Check sheet for the modelled part. Datum: model origin and axes. Units: mm. Give positions to 0.01 mm unless a question says otherwise; leave off trailing zeros. Order: outer loops, then holes, each group sorted by start corner. A loop starts at its lowest first (then second) coordinate and runs counter-clockwise, first axis right, second up. Notation, with made-up numbers: (-34, -37) -> (18, -37) arc R7 ccw to (18, -29) -> close; hole circle Ø5 at (20, 74.5). An arc over 180 degrees is marked (long way). Answer in a Markdown table with one row per item. Add a question column.
(1) Cross-section at A-A (z = 3.8). State how many separate pieces and enclosed holes the cut face has, then the cut area to 3 significant figures.
(2) Cross-section at D-D (x = 42). Record the cut outline in (y, z).
(3) Thickness scan on L1, parallel to Y at x = 71, z = 1.25; L2, parallel to Z at x = 111.5, y = -42.75; L3, parallel to Y at x = 30, z = 3.4. Record the ranges inside material, lowest first. Write a range as [from, to].
(4) Go/stop test with flat-tipped pins: pin 1 (2.5 mm diameter, centred on x = 157.5, z = 2, fed in from -Y); pin 2 (0.9 mm diameter, centred on x = 23.5, y = -42, fed in from +Z); pin 3 (1 mm diameter, centred on x = 101.5, z = 4, fed in from +Y). Record where each tip stops, or that it passes through.
(5) Cross-section at B-B (x = 102). Record the cut outline in (y, z), then the cut area to 3 significant figures.
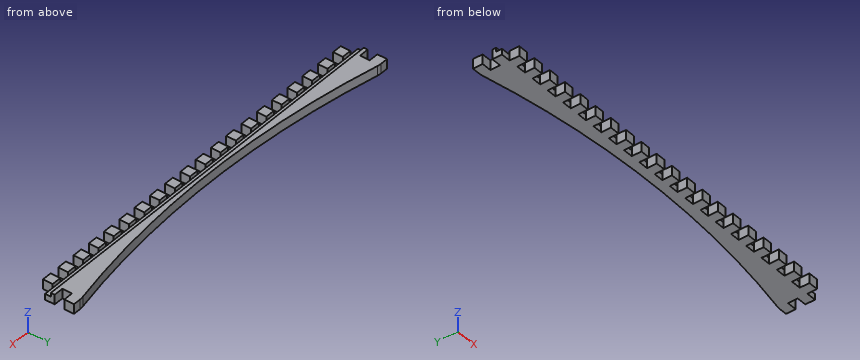
```python
from build123d import *

# Parameters (mm, degrees)
ESQUISSE1_W             = 205
ESQUISSE1_H             = 20
BOSS_EXTRU_1_DEPTH      = 5
ESQUISSE2_W             = 5
ESQUISSE2_H             = 5
ENL_V_MAT_EXTRU_2_DEPTH = 5
ESQUISSE3_W             = 205
ESQUISSE3_H             = 3
ENL_V_MAT_EXTRU_3_DEPTH = 2
CONG_2_R                = 10
CONG_3_R                = 10


with BuildPart() as part:
    # Esquisse1 → Boss.-Extru.1 (new body)
    with BuildSketch(Plane.XY):
        with Locations((56.490511124, -39.453030303)):
            Rectangle(ESQUISSE1_W, ESQUISSE1_H)
    extrude(amount=BOSS_EXTRU_1_DEPTH)

    # Esquisse2 → Enlèv. mat.-Extru.2 (cut)
    with BuildSketch(Plane.XY.offset(5)):
        with Locations((146.490511124, -46.953030303)):
            Rectangle(ESQUISSE2_W, ESQUISSE2_H)
        with Locations((156.490511124, -46.953030303)):
            Rectangle(ESQUISSE2_W, ESQUISSE2_H)
        with Locations((136.490511124, -46.953030303)):
            Rectangle(ESQUISSE2_W, ESQUISSE2_H)
        with Locations((126.490511124, -46.953030303)):
            Rectangle(ESQUISSE2_W, ESQUISSE2_H)
        with Locations((116.490511124, -46.953030303)):
            Rectangle(ESQUISSE2_W, ESQUISSE2_H)
        with Locations((106.490511124, -46.953030303)):
            Rectangle(ESQUISSE2_W, ESQUISSE2_H)
        with Locations((96.490511124, -46.953030303)):
            Rectangle(ESQUISSE2_W, ESQUISSE2_H)
        with Locations((86.490511124, -46.953030303)):
            Rectangle(ESQUISSE2_W, ESQUISSE2_H)
        with Locations((76.490511124, -46.953030303)):
            Rectangle(ESQUISSE2_W, ESQUISSE2_H)
        with Locations((66.490511124, -46.953030303)):
            Rectangle(ESQUISSE2_W, ESQUISSE2_H)
        with Locations((56.490511124, -46.953030303)):
            Rectangle(ESQUISSE2_W, ESQUISSE2_H)
        with Locations((46.490511124, -46.953030303)):
            Rectangle(ESQUISSE2_W, ESQUISSE2_H)
        with Locations((36.490511124, -46.953030303)):
            Rectangle(ESQUISSE2_W, ESQUISSE2_H)
        with Locations((26.490511124, -46.953030303)):
            Rectangle(ESQUISSE2_W, ESQUISSE2_H)
        with Locations((16.490511124, -46.953030303)):
            Rectangle(ESQUISSE2_W, ESQUISSE2_H)
        with Locations((6.490511124, -46.953030303)):
            Rectangle(ESQUISSE2_W, ESQUISSE2_H)
        with Locations((-3.509488876, -46.953030303)):
            Rectangle(ESQUISSE2_W, ESQUISSE2_H)
        with Locations((-13.509488876, -46.953030303)):
            Rectangle(ESQUISSE2_W, ESQUISSE2_H)
        with Locations((-23.509488876, -46.953030303)):
            Rectangle(ESQUISSE2_W, ESQUISSE2_H)
        with Locations((-33.509488876, -46.953030303)):
            Rectangle(ESQUISSE2_W, ESQUISSE2_H)
        with Locations((156.490511124, -36.953030303)):
            Rectangle(ESQUISSE2_W, ESQUISSE2_H)
        with BuildLine():
            Line((-41.009488876, -29.453030303), (153.990511124, -29.453030303))
            ThreePointArc((153.990511124, -29.453030303), (56.490511124, -39.694920166), (-41.009488876, -29.453030303))
        make_face()
        with Locations((-43.509488876, -46.953030303)):
            Rectangle(ESQUISSE2_W, ESQUISSE2_H)
        with Locations((-43.509488876, -36.953030303)):
            Rectangle(ESQUISSE2_W, ESQUISSE2_H)
    extrude(amount=-ENL_V_MAT_EXTRU_2_DEPTH, mode=Mode.SUBTRACT)

    # Esquisse3 → Enlèv. mat.-Extru.3 (cut)
    with BuildSketch(Plane.XY.offset(5)):
        with Locations((56.490511124, -42.953030303)):
            Rectangle(ESQUISSE3_W, ESQUISSE3_H)
    extrude(amount=-ENL_V_MAT_EXTRU_3_DEPTH, mode=Mode.SUBTRACT)

    # Congé2
    cong_2_edges = [part.edges().sort_by_distance(p)[0] for p in [
        (153.990511124, -29.453030303, 2.5),
    ]]
    fillet(cong_2_edges, radius=CONG_2_R)

    # Congé3
    cong_3_edges = [part.edges().sort_by_distance(p)[0] for p in [
        (-41.009488876, -29.453030303, 2.5),
    ]]
    fillet(cong_3_edges, radius=CONG_3_R)


solid = part.part
```
Answer below:
| question | item | result |
|---|---|---|
| 1 | separate pieces | 21 |
| 1 | enclosed holes | 0 |
| 1 | area | 1,580 mm² |
| 2 | outline | (-49.45, 0) -> (-39.47, 0) -> (-39.47, 5) -> (-41.45, 5) -> (-41.45, 3) -> (-44.45, 3) -> (-44.45, 5) -> (-49.45, 5) -> close |
| 3 | L1 | y = [-49.45, -39.47] |
| 3 | L2 | z = [0, 3] |
| 3 | L3 | y = [-49.45, -44.45], [-41.45, -38.95] |
| 4 | pin 1 | stops at y = -44.45 |
| 4 | pin 2 | stops at z = 3 |
| 4 | pin 3 | stops at y = -37.48 |
| 5 | outline | (-49.45, 0) -> (-37.48, 0) -> (-37.48, 5) -> (-41.45, 5) -> (-41.45, 3) -> (-44.45, 3) -> (-44.45, 5) -> (-49.45, 5) -> close |
| 5 | area | 53.9 mm² |
